For this review, use the dimensioned drawing (mm, ordinates from the lowest corner) and the shaded views. A direction names the side the tool comes from. Give positions to 0.01 mm unless a question says otherwise; leave off trailing zeros. Order: outer loops, then holes, each group sorted by start corner. A loop starts at its lowest first (then second) coordinate and runs counter-clockwise, first axis right, second up. Notation, with made-up numbers: M 59.25,33 L 79.25,33 A30 ccw 79.25,65 Z; hole C 22,45 d10. An arc over 180 degrees is marked long. Use CSV: the item, a comma, the result in double quotes. Start each with the question number.
(1) Consider section B-B (z = 4). Write out the cut boundary in (x, y), and give its area (3 significant figures).
(2) Consider section A-A (y = 19). Give the number of separate pieces and of enclosed holes in the cut face, and give its area (3 significant figures).
(3) Consider section D-D (z = 40). Write out the cut boundary in (x, y), and give its area (3 significant figures).
(4) Draft analysis for pull direction X (two halves, no side actions). For the marked faces 3, 4 and 5, state which applies: pulls with the +X half, pulls with the -X half, needs draft (parallel to the pull), parting line crosses it, or undercut.
(5) Clearance check with flat-ended pins moving along their axes: P1, Ø2, axis at x = 11, z = 8, coming from the +Y side; P2, Ø3, axis at x = 25.5, z = 64, coming from the -Y side; P3, Ø0.5, axis at x = 59, z = 64, coming from the +Y side. State where each tip first meets the part, or that it passes through.
(6) Tool access review of the marked faces 1 and 2: name each direction out of +Z, -Z, +X, -X, +Y, -Y from which nothing blocks a thin tool from reaching the whole face with its end or side.
(7) Wall thickness on L1, parallel to Y at x = 1.8, z = 4; L2, parallel to X at y = 23.5, z = 66.5; L3, parallel to Z at x = 76.5, y = 27: over which ranges is each line inside the solid? List them lowest first. Write a range as from..to.
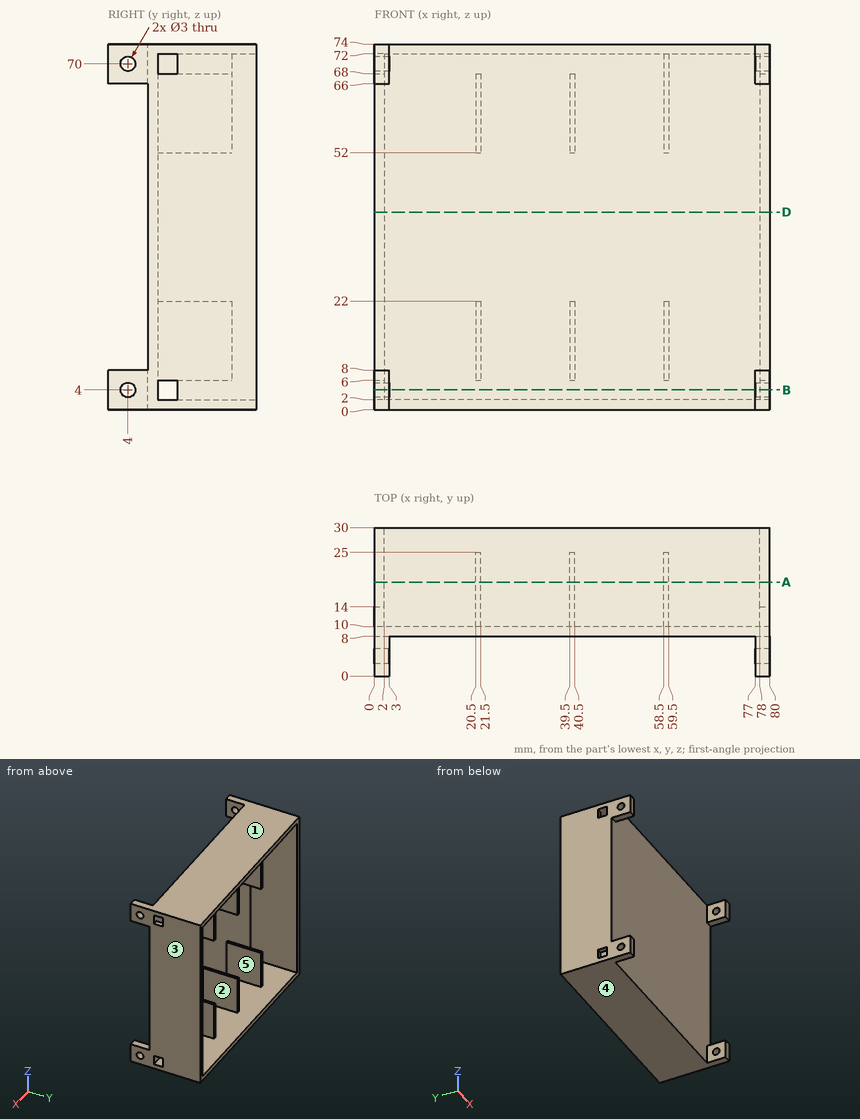
Check result:
1,outline,"M 0,0 L 3,0 L 3,2.5 L 0,2.5 Z; M 0,5.5 L 3,5.5 L 3,8 L 77,8 L 77,5.5 L 80,5.5 L 80,10 L 0,10 Z; M 0,14 L 2,14 L 2,30 L 0,30 Z; M 77,0 L 80,0 L 80,2.5 L 77,2.5 Z; M 78,14 L 80,14 L 80,30 L 78,30 Z"
1,area,"254 mm^2"
2,separate pieces,"6"
2,enclosed holes,"1"
2,area,"700 mm^2"
3,outline,"M 0,8 L 80,8 L 80,30 L 78,30 L 78,10 L 2,10 L 2,30 L 0,30 Z"
3,area,"240 mm^2"
4,face 3,"pulls with the +X half"
4,face 4,"needs draft"
4,face 5,"undercut"
5,P1,"stops at y = 10"
5,P2,"stops at y = 8"
5,P3,"stops at y = 25"
6,face 1,"+Z, +X, -X, +Y, -Y"
6,face 2,"+Y"
7,L1,"y = 0..2.5, 5.5..10, 14..30"
7,L2,"x = 0..2, 20.5..21.5, 39.5..40.5, 58.5..59.5, 78..80"
7,L3,"z = 0..2, 72..74"
